```python
from build123d import *

# Parameters (mm, degrees)
BOSS_EXTRUDE1_DEPTH   = 45
CUT_EXTRUDE1_START    = -5
CUT_EXTRUDE1_DEPTH    = 2
M4X0_7_TAPPED_HOLE1_D = 3.3
SKETCH5_R             = 7.5
BOSS_EXTRUDE2_DEPTH   = 45
SKETCH6_R             = 3.875
CUT_EXTRUDE2_DEPTH    = 46


with BuildPart() as part:
    # Sketch1 → Boss-Extrude1 (new body)
    with BuildSketch(Plane.XY):
        with BuildLine():
            Line((-182.516015687, 162.517772537), (-174, 161.93046111))
            Line((-174, 161.93046111), (-174, 141.5))
            Line((-174, 141.5), (-161, 141.5))
            Line((-161, 141.5), (-161, 176.06953889))
            Line((-161, 176.06953889), (-181.483984313, 177.482227463))
            ThreePointArc((-181.483984313, 177.482227463), (-174.517772537, 169.483984313), (-182.516015687, 162.517772537))
        make_face()
    extrude(amount=BOSS_EXTRUDE1_DEPTH)

    # Sketch2 → Cut-Extrude1 (cut, symmetric)
    with BuildSketch(Plane(origin=(0, 0, 0), x_dir=(-1, 0, 0), z_dir=(0, 0, -1)).offset(CUT_EXTRUDE1_START)):
        with BuildLine():
            ThreePointArc((176.520836095, 177.139941379), (173.021327044, 169.380781175), (177.552867469, 162.175486453))
            ThreePointArc((177.552867469, 162.175486453), (177.834315887, 161.15284928), (176.811678714, 160.871400862))
            ThreePointArc((176.811678714, 160.871400862), (171.524881552, 169.277578038), (175.60764211, 178.329931609))
            ThreePointArc((175.60764211, 178.329931609), (176.659234217, 178.191533486), (176.520836095, 177.139941379))
        make_face()
    cut_extrude1 = extrude(amount=CUT_EXTRUDE1_DEPTH, both=True, mode=Mode.SUBTRACT)

    # Mirror1: Cut-Extrude1 across plane
    add(cut_extrude1.mirror(Plane(origin=(0, 0, 22.5), x_dir=(1, 0, 0), z_dir=(0, 0, -1))), mode=Mode.SUBTRACT)

    # M4x0.7 Tapped Hole1 (through all)
    with Locations(Plane.XY.offset(45)):
        with Locations((-167.5, 169), (-167.5, 146.5)):
            Hole(M4X0_7_TAPPED_HOLE1_D / 2)

    # Sketch5 → Boss-Extrude2 (add, through all)
    with BuildSketch(Plane.XY.offset(45)):
        with Locations((-182, 170)):
            Circle(SKETCH5_R)
    extrude(amount=-BOSS_EXTRUDE2_DEPTH)

    # Sketch6 → Cut-Extrude2 (cut, through all)
    with BuildSketch(Plane.XY.offset(45)):
        with Locations((-182, 170)):
            Circle(SKETCH6_R)
    extrude(amount=-CUT_EXTRUDE2_DEPTH, mode=Mode.SUBTRACT)

    # Sketch9 → Cut-Revolve1 (revolve, cut)
    with BuildSketch(Plane(origin=(10.807100592, 156.70295858, 0), x_dir=(-0.997630328, 0.068802092, 0), z_dir=(-0.068802092, -0.997630328, 0))):
        Polygon((189.390075348, -9), (187.890075348, -12.5), (189.390075348, -16), align=None)
        Polygon((189.390075348, -19), (189.390075348, -26), (187.890075348, -22.5), align=None)
        Polygon((189.390075348, -29), (189.390075348, -36), (187.890075348, -32.5), align=None)
    revolve(axis=Axis((-182, 170, 0), (0, 0, 1)), mode=Mode.SUBTRACT)


solid = part.part
```
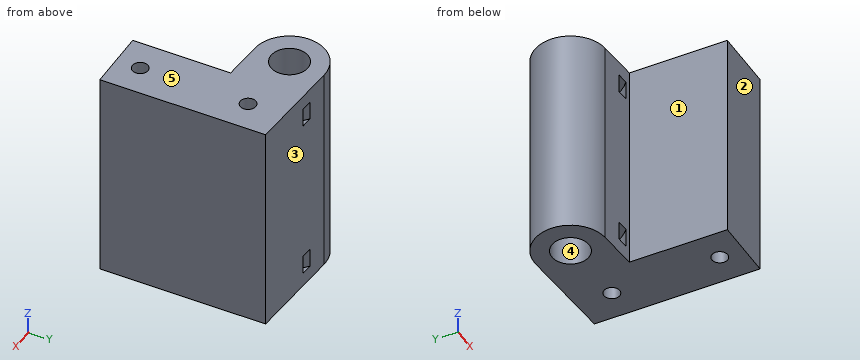
Here's how the part is built. I have some questions about the finished solid (model axes, mm). Face numbers are marked on the shaded views. A direction names the side the tool comes from. Coordinates: 2 decimals unless noted, no trailing zeros. Order: outer loops, then holes, each group sorted by start corner. A loop starts at its lowest first (then second) coordinate and runs counter-clockwise, first axis right, second up. Notation, with made-up numbers: (61.5, 22.25) -> (118.5, 22.25) arc R13 ccw to (118.5, 29.25) -> close; hole circle Ø11 at (64.5, 49.25). An arc over 180 degrees is marked (long way). Return JSON: item names as keys, results as strings.
1) If I drill on probe 1 along Z at (x, y) = (-175.25, 176); probe 2 along X at (y, z) = (170, 6) (3 decimals); probe 3 along X at (y, z) = (169, 23.5), over which ranges is the centre line in solid material (lowest first)?
Conclusion:
{"probe 1": "z = 0 to 3, 7 to 38, 42 to 45", "probe 2": "x = -189.5 to -185.875, -178.125 to -173, -171.5 to -168.812, -166.188 to -161", "probe 3": "x = -189.43 to -186.84, -177.16 to -169.15, -165.85 to -161"}
2) On a 3-axis mill with a long thin cutter (end or side, diameter ignored), from which of +Z, -Z, +X, -X, +Y, -Y can I reach the whole of each face in a straight line? I mean the marked faces 1 and 2. Say none if no direction works.
Conclusion:
{"face 1": "+Z, -Z, -X, -Y", "face 2": "+Z, -Z, +X, -X, -Y"}
3) If we section it at C-C on x = -166.75: List the corners of the cut face in (y, z) for me, plus the area to 3 significant figures.
Conclusion:
{"outline": "(141.5, 0) -> (145.03, 0) -> (145.03, 45) -> (141.5, 45) -> close; (147.97, 0) -> (167.53, 0) -> (167.53, 45) -> (147.97, 45) -> close; (170.47, 0) -> (176.47, 0) -> (176.47, 45) -> (170.47, 45) -> close", "area": "1,310 mm²"}
4) If we section it at D-D on z = 5: List the corners of the cut face in (x, y) for me (3 decimals), plus the area to 3 significant figures.
Conclusion:
{"outline": "(-182.516, 162.518) -> (-177.553, 162.175) arc R9 ccw to (-176.521, 177.14) -> (-181.484, 177.482) arc R7.5 ccw to start; (-175.185, 162.012) -> (-174, 161.93) -> (-174, 141.5) -> (-161, 141.5) -> (-161, 176.07) -> (-174.153, 176.977) arc R10.5 cw to start; hole circle Ø7.75 at (-182, 170); hole circle Ø3.3 at (-167.5, 146.5); hole circle Ø3.3 at (-167.5, 169)", "area": "574 mm²"}
5) Thinking about a two-plate mould opening in X: for the marked faces 3, 4 and 5, which applies, +X half, -X half, draft (parallel to the pull), parting line (faces both ways), or undercut?
Conclusion:
{"face 3": "+X half", "face 4": "undercut", "face 5": "draft"}
6) If we section it at B-B on z = 28: List the corners of the cut face in (x, y) for me (3 decimals).
Conclusion:
{"outline": "(-182.516, 162.518) -> (-174, 161.93) -> (-174, 141.5) -> (-161, 141.5) -> (-161, 176.07) -> (-181.484, 177.482) arc R7.5 ccw to start; hole circle Ø7.75 at (-182, 170); hole circle Ø3.3 at (-167.5, 146.5); hole circle Ø3.3 at (-167.5, 169)"}
7) I'm going to push flat-ended pins straight in: P1, Ø12, axis at x = -172.5, z = 16, coming from the +Y side; P2, Ø3, axis at y = 151.5, z = 19, coming from the -X side; P3, Ø1.5, axis at x = -182, z = 27, coming from the -Y side; P4, Ø2, axis at x = -167.5, y = 169, coming from the +Z side. Where does each tip first touch, or does it pass through?
Conclusion:
{"P1": "stops at y = 177.28", "P2": "stops at x = -174", "P3": "stops at y = 162.43", "P4": "passes through"}
8) If we section it at A-A on y = 146.5: List the corners of the cut face in (x, z) for me, plus the area to 4 significant figures.
Conclusion:
{"outline": "(-174, 0) -> (-169.15, 0) -> (-169.15, 45) -> (-174, 45) -> close; (-165.85, 0) -> (-161, 0) -> (-161, 45) -> (-165.85, 45) -> close", "area": "436.5 mm²"}
